For this review, use the dimensioned drawing (mm, ordinates from the lowest corner) and the shaded views. A direction names the side the tool comes from. Coordinates: 2 decimals unless noted, no trailing zeros. Write each loop counter-clockwise with the first axis right and the second up, starting at its lowest first coordinate (ties: lowest second). Pieces come first, ordered by that corner, then holes. Notation, with made-up numbers: (-11.5, 40.25) - (34.5, 40.25) arc R34 ccw to (34.5, 78.25) - close; hole circle Ø3 at (-32.75, 50.5). An arc over 180 degrees is marked (long way). Use one line per item in the form item = value. Start each with the question number.
1) Insertion check: P1, Ø12, axis at x = 21.5, z = 27, coming from the -Y side; P2, Ø2.5, axis at x = 35.15, z = 41.62, coming from the -Y side. Each pin has a flat end and moves straight along its axis. Give the tip position at first contact, or say it passes through.
2) We need section C-C (y = 18). Give the boundary of the cut face in (x, z).
3) We need section A-A (z = 12.5). Give the boundary of the cut face in (x, y).
4) We need section B-B (x = 19). Give the boundary of the cut face in (y, z), plus the area to 3 significant figures.
5) Tool access review of the marked faces 1 and 2: name each direction out of +Z, -Z, +X, -X, +Y, -Y from which nothing blocks a thin tool from reaching the whole face with its end or side.
6) For L1, parallel to Y at x = 4, z = 28; L2, parallel to Y at x = 19, z = 48.4; L3, parallel to Z at x = 12, y = 5.5, list the stretches that pass through material, from the lowest coordinate up. Write a range as from..to.
7) Mouldability with a two-part tool opening along Y and no side actions: class the marked faces 3, 4, 5 and 6 as pulls with the +Y half, pulls with the -Y half, needs draft (parallel to the pull), parting line crosses it, or undercut.
8) We need section D-D (y = 3). Give the boundary of the cut face in (x, z), plus the area to 3 significant figures.
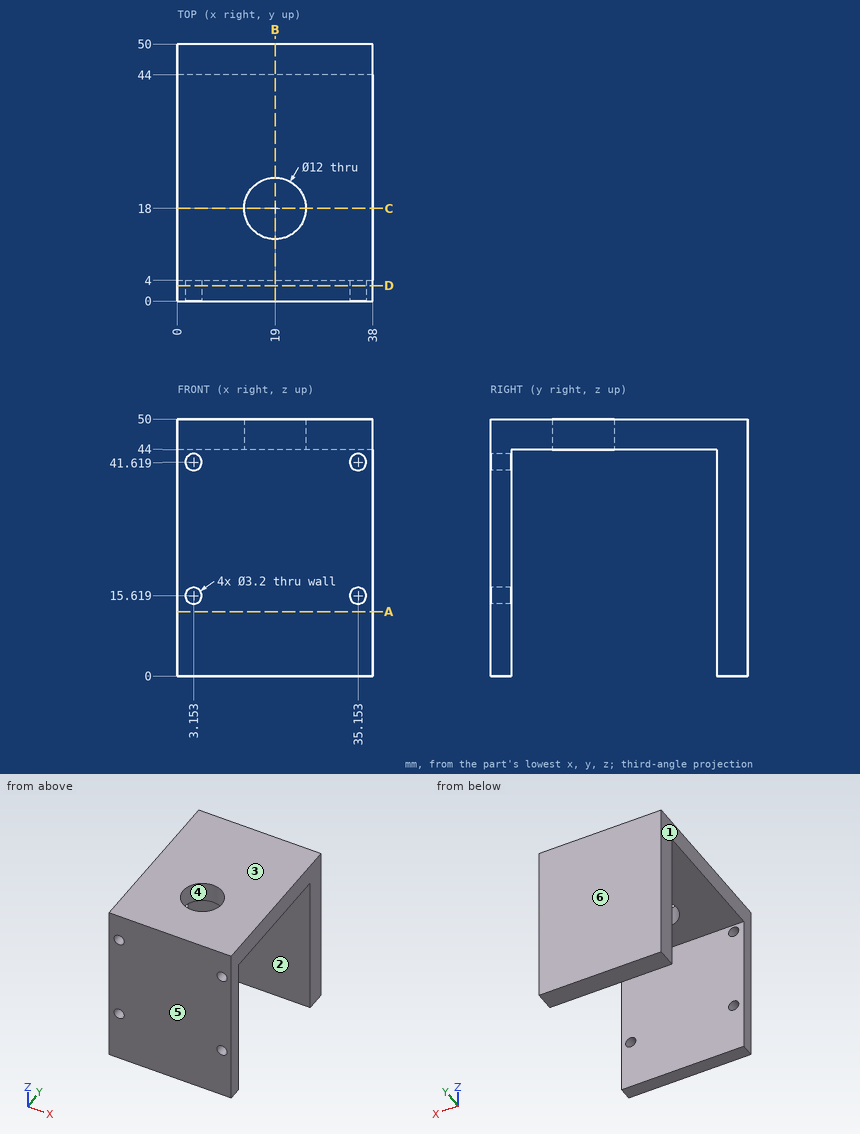
Determined:
q1.P1 = 0
q1.P2 = 44
q2.outline = (0, 44) - (13, 44) - (13, 50) - (0, 50) - close; (25, 44) - (38, 44) - (38, 50) - (25, 50) - close
q3.outline = (0, 0) - (38, 0) - (38, 4) - (0, 4) - close; (0, 44) - (38, 44) - (38, 50) - (0, 50) - close
q4.outline = (0, 0) - (4, 0) - (4, 44) - (12, 44) - (12, 50) - (0, 50) - close; (24, 44) - (44, 44) - (44, 0) - (50, 0) - (50, 50) - (24, 50) - close
q4.area = 668 mm²
q5.face_1 = +Z, -Z, -X, +Y, -Y
q5.face_2 = -Z, +X, -X
q6.L1 = 0..4, 44..50
q6.L2 = 0..12, 24..50
q6.L3 = 44..50
q7.face_3 = needs draft
q7.face_4 = undercut
q7.face_5 = pulls with the -Y half
q7.face_6 = pulls with the +Y half
q8.outline = (0, 0) - (38, 0) - (38, 50) - (0, 50) - close; hole circle Ø3.2 at (3.15, 15.62); hole circle Ø3.2 at (3.15, 41.62); hole circle Ø3.2 at (35.15, 15.62); hole circle Ø3.2 at (35.15, 41.62)
q8.area = 1,870 mm²
